Print and shaded views of the part. All mm, measured from the part's lowest x, y and z. A direction names the side the tool comes from. Round coordinates to 2 decimals unless told otherwise and drop trailing zeros. Loops run counter-clockwise (first coordinate to the right, second up) from the corner with the lowest first, then second, coordinate; pieces in that order, holes last. Notation, with made-up numbers: (-29, 75) -> (-8, 75) arc R26 ccw to (-8, 95) -> close; hole circle Ø8 at (31.5, 89). An arc over 180 degrees is marked (long way). Use a Markdown table: item, result.
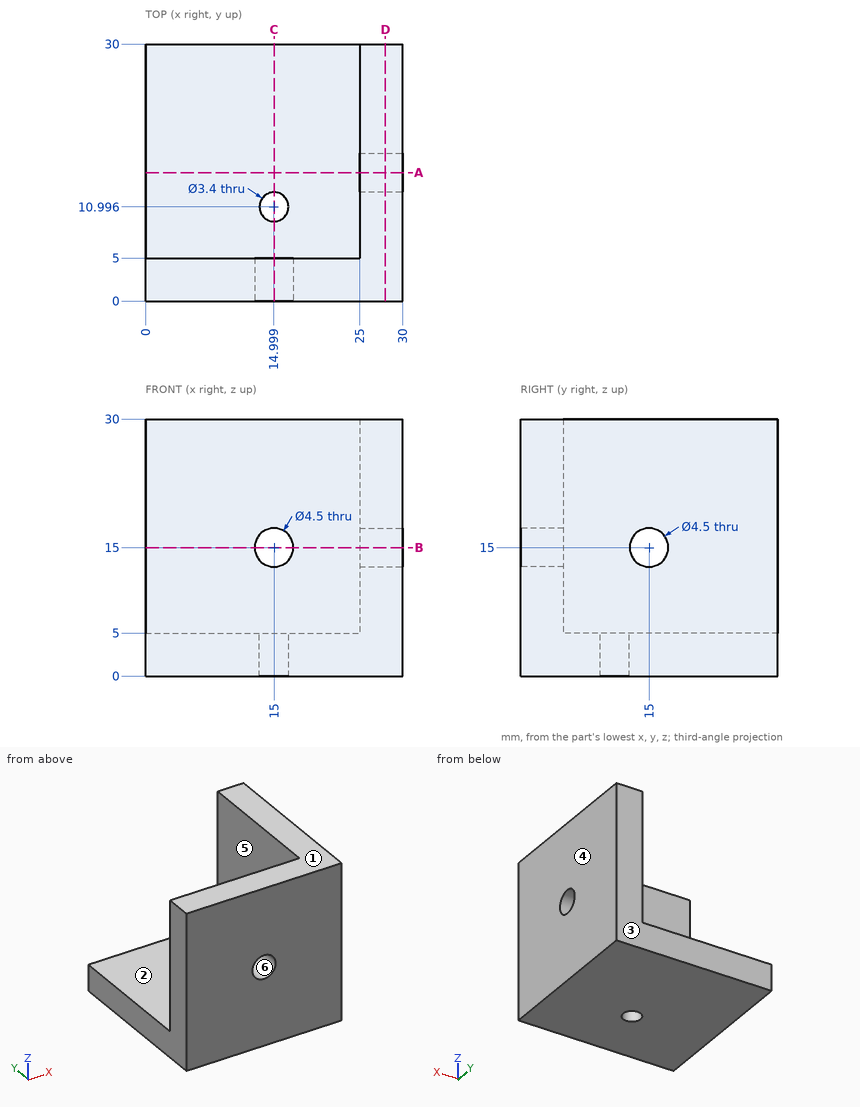
Q1. Band-saw the part on D-D, the plane x = 28. Give the cut face in (y, z).
Results list:
| item | result |
|---|---|
| outline | (0, 0) -> (30, 0) -> (30, 30) -> (0, 30) -> close; hole circle Ø4.5 at (15, 15) |
Q2. Drill centre lines: L1, parallel to X at y = 2, z = 15; L2, parallel to Y at x = 13.5, z = 22.75. Where is each one in solid material? Low to high. Write a range as from..to.
Results list:
| item | result |
|---|---|
| L1 | x = 0..12.75, 17.25..30 |
| L2 | y = 0..5 |
Q3. Band-saw the part on B-B, the plane z = 15. Give the cut face in (x, y).
Results list:
| item | result |
|---|---|
| outline | (0, 0) -> (12.75, 0) -> (12.75, 5) -> (0, 5) -> close; (17.25, 0) -> (30, 0) -> (30, 12.75) -> (25, 12.75) -> (25, 5) -> (17.25, 5) -> close; (25, 17.25) -> (30, 17.25) -> (30, 30) -> (25, 30) -> close |
Q4. Band-saw the part on A-A, the plane y = 15. Give the cut face in (x, z).
Results list:
| item | result |
|---|---|
| outline | (0, 0) -> (30, 0) -> (30, 12.75) -> (25, 12.75) -> (25, 5) -> (0, 5) -> close; (25, 17.25) -> (30, 17.25) -> (30, 30) -> (25, 30) -> close |
Q5. Tool access for the marked faces 1 and 2: list every direction of +Z, -Z, +X, -X, +Y, -Y with a clear straight run to the whole face (end or side of a thin tool).
Results list:
| item | result |
|---|---|
| face 1 | +Z, +X, -X, +Y, -Y |
| face 2 | +Z, -X, +Y |
Q6. Band-saw the part on C-C, the plane x = 15. Give the cut face in (y, z).
Results list:
| item | result |
|---|---|
| outline | (0, 0) -> (9.3, 0) -> (9.3, 5) -> (5, 5) -> (5, 12.75) -> (0, 12.75) -> close; (0, 17.25) -> (5, 17.25) -> (5, 30) -> (0, 30) -> close; (12.7, 0) -> (30, 0) -> (30, 5) -> (12.7, 5) -> close |
Q7. Pull direction X, two halves, no side cores. Call the marked faces 3, 4, 5 and 6: released by +X, released by -X, zero draft, split by the parting line, or undercut.
Results list:
| item | result |
|---|---|
| face 3 | zero draft |
| face 4 | released by +X |
| face 5 | released by -X |
| face 6 | undercut |
Q8. Flat gauge pins, fed straight in: pin 1 (12 mm diameter, centred on x = 9, y = 26, fed in from -Z); pin 2 (10 mm diameter, centred on y = 13.5, z = 20, fed in from -X); pin 3 (4 mm diameter, centred on x = 14, z = 15.5, fed in from +Y); pin 4 (4 mm diameter, centred on x = 13.5, y = 8.5, fed in from +Z). Where does each tip first touch, or does it go through?
Results list:
| item | result |
|---|---|
| pin 1 | stops at z = 0 |
| pin 2 | stops at x = 25 |
| pin 3 | stops at y = 5 |
| pin 4 | stops at z = 5 |
